Check sheet for the modelled part. Datum: model origin and axes. Units: mm. Round coordinates to 2 decimals unless told otherwise and drop trailing zeros. Order: outer loops, then holes, each group sorted by start corner. A loop starts at its lowest first (then second) coordinate and runs counter-clockwise, first axis right, second up. Notation, with made-up numbers: (25, -31.75) -> (29, -31.75) arc R24 cw to (29, -5.75) -> close; hole circle Ø6 at (-17, 29). An arc over 180 degrees is marked (long way). Answer in a Markdown table with one row per item.
```python
from build123d import *

# Parameters (mm, degrees)
SKETCH1_R           = 11
BOSS_EXTRUDE1_DEPTH = 4
SKETCH2_R           = 5.15
BOSS_EXTRUDE2_DEPTH = 11
SKETCH3_R           = 4
CUT_EXTRUDE1_DEPTH  = 16
SKETCH4_R           = 1.5
CUT_EXTRUDE2_DEPTH  = 5


with BuildPart() as part:
    # Sketch1 → Boss-Extrude1 (new body)
    with BuildSketch(Plane.XY):
        Circle(SKETCH1_R)
    extrude(amount=BOSS_EXTRUDE1_DEPTH)

    # Sketch2 → Boss-Extrude2 (add)
    with BuildSketch(Plane.XY.offset(4)):
        Circle(SKETCH2_R)
    extrude(amount=BOSS_EXTRUDE2_DEPTH)

    # Sketch3 → Cut-Extrude1 (cut, through all)
    with BuildSketch(Plane.XY.offset(15)):
        Circle(SKETCH3_R)
    extrude(amount=-CUT_EXTRUDE1_DEPTH, mode=Mode.SUBTRACT)

    # Sketch4 → Cut-Extrude2 (cut, through all)
    with BuildSketch(Plane.XY.offset(4)):
        with Locations((0, 8)):
            Circle(SKETCH4_R)
        with Locations((8, 0)):
            Circle(SKETCH4_R)
        with Locations((0, -8)):
            Circle(SKETCH4_R)
        with Locations((-8, 0)):
            Circle(SKETCH4_R)
    extrude(amount=-CUT_EXTRUDE2_DEPTH, mode=Mode.SUBTRACT)


solid = part.part
```
(1) Draft check along X on faces 1 (the cylindrical face through (-0.867, -3.905, 7.605)), 2 (the flat face through (2, -5, 4)), 3 (the cylindrical face through (4.91, 1.55, 9.42)). Enter one of: pulls with the +X half, pulls with the -X half, needs draft (parallel to the pull), parting line crosses it, or undercut.
Solutions:
| item | result |
|---|---|
| face 1 | undercut |
| face 2 | needs draft |
| face 3 | parting line crosses it |
(2) Scan lines: probe 1 along Y at (x, z) = (0, 1.6); probe 2 along Y at (x, z) = (0, 8); probe 3 along Y at (x, z) = (0.5, 2.75). Record each from-to range of solid material in increasing order. Write a range as from..to.
Solutions:
| item | result |
|---|---|
| probe 1 | -11..-9.5, -6.5..-4, 4..6.5, 9.5..11 |
| probe 2 | -5.15..-4, 4..5.15 |
| probe 3 | -10.99..-9.41, -6.59..-3.97, 3.97..6.59, 9.41..10.99 |
(3) Section check A-A on x = 0. Record the boundary of the cut face in (y, z).
Solutions:
| item | result |
|---|---|
| outline | (-11, 0) -> (-9.5, 0) -> (-9.5, 4) -> (-11, 4) -> close; (-6.5, 0) -> (-4, 0) -> (-4, 15) -> (-5.15, 15) -> (-5.15, 4) -> (-6.5, 4) -> close; (4, 0) -> (6.5, 0) -> (6.5, 4) -> (5.15, 4) -> (5.15, 15) -> (4, 15) -> close; (9.5, 0) -> (11, 0) -> (11, 4) -> (9.5, 4) -> close |
(4) Section check C-C on z = 3. Record the boundary of the cut face in (x, y), plus the area to 3 significant figures.
Solutions:
| item | result |
|---|---|
| outline | circle Ø22 at (0, 0); hole circle Ø3 at (-8, 0); hole circle Ø8 at (0, 0); hole circle Ø3 at (0, -8); hole circle Ø3 at (0, 8); hole circle Ø3 at (8, 0) |
| area | 302 mm^2 |
(5) Section check D-D on x = -8. Record the boundary of the cut face in (y, z), plus the area to 3 significant figures.
Solutions:
| item | result |
|---|---|
| outline | (-7.55, 0) -> (-1.5, 0) -> (-1.5, 4) -> (-7.55, 4) -> close; (1.5, 0) -> (7.55, 0) -> (7.55, 4) -> (1.5, 4) -> close |
| area | 48.4 mm^2 |
(6) Depth check by flat-ended pin: pin 1 Ø1.5 at (x, z) = (1.5, 8.5) entering from +Y; pin 2 Ø2.5 at (x, y) = (0, -8) entering from +Z; pin 3 Ø1.5 at (x, y) = (1, -8.5) entering from +Z; pin 4 Ø1.5 at (y, z) = (-1.5, 12) entering from +X. Enter the tip coordinate at first touch or a pass-through.
Solutions:
| item | result |
|---|---|
| pin 1 | y = 5.1 |
| pin 2 | through |
| pin 3 | z = 4 |
| pin 4 | x = 5.1 |
